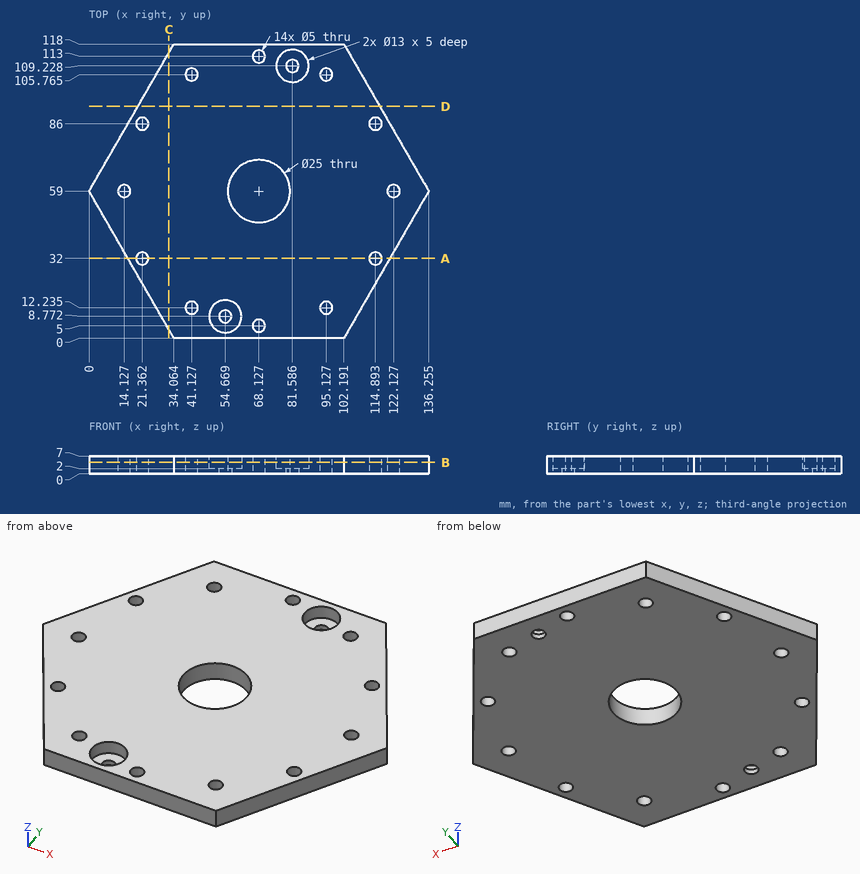
The drawing under review shows one solid part. Ordinate dimensions are in mm from its lowest x, y, z. Coordinates: 2 decimals unless noted, no trailing zeros. Order: outer loops, then holes, each group sorted by start corner. A loop starts at its lowest first (then second) coordinate and runs counter-clockwise, first axis right, second up. Notation, with made-up numbers: (40, 81.25) -> (66, 81.25) arc R20 cw to (66, 119.25) -> close; hole circle Ø11 at (15, 75.5). An arc over 180 degrees is marked (long way). Return JSON: item names as keys, results as strings.
1. For line 1 (Y direction, x = 96, z = 4.75); line 2 (X direction, y = 107, z = 3.75) (1 decimal); line 3 (Y direction, x = 43, z = 1), list the stretches that pass through material, from the lowest coordinate up. Write a range as from..to.
Answer block:
{"line 1": "0..9.89, 14.58..103.42, 108.11..118", "line 2": "27.7..39, 43.3..75.5, 87.7..93, 97.3..108.5", "line 3": "0..10.58, 13.89..104.11, 107.42..118"}
2. We need section D-D on y = 93. Write out the cut boundary in (x, z) (1 decimal).
Answer block:
{"outline": "(19.6, 0) -> (116.6, 0) -> (116.6, 7) -> (19.6, 7) -> close"}
3. We need section B-B on z = 4.5. State how many separate pieces and enclosed holes the cut face has, and give its area (3 significant figures).
Answer block:
{"separate pieces": "1", "enclosed holes": "15", "area": "11,100 mm²"}
4. We need section A-A on y = 32. Write out the cut boundary in (x, z).
Answer block:
{"outline": "(15.59, 0) -> (18.86, 0) -> (18.86, 7) -> (15.59, 7) -> close; (23.86, 0) -> (112.39, 0) -> (112.39, 7) -> (23.86, 7) -> close; (117.39, 0) -> (120.67, 0) -> (120.67, 7) -> (117.39, 7) -> close"}
5. For pin 1 Ø3 at (y, z) = (55.5, 6) entering from -X (1 decimal); pin 2 Ø1 at (x, y) = (112, 41.5) entering from -Z; pin 3 Ø4 at (x, y) = (114.89, 32) entering from +Z; pin 4 Ø8 at (x, y) = (54.67, 8.77) entering from +Z, all flat-tipped, find the tip position at first contact; note any pin that passes through.
Answer block:
{"pin 1": "x = 1.2", "pin 2": "z = 0", "pin 3": "through", "pin 4": "z = 2"}
6. We need section C-C on x = 32. Write out the cut boundary in (y, z) (1 decimal).
Answer block:
{"outline": "(3.6, 0) -> (114.4, 0) -> (114.4, 7) -> (3.6, 7) -> close"}
